```python
from build123d import *

# Parameters (mm, degrees)
SKETCH1_W                      = 95
SKETCH1_H                      = 34
BOSS_EXTRUDE1_DEPTH            = 6.5
SKETCH2_W                      = 74
SKETCH2_H                      = 5
BOSS_EXTRUDE2_DEPTH            = 90
SKETCH3_W                      = 58
SKETCH3_H                      = 22
CUT_EXTRUDE1_DEPTH             = 90
CBORE_FOR_M3_SHCS1_D           = 3.4
CBORE_FOR_M3_SHCS1_DEPTH       = 10.1
CBORE_FOR_M3_SHCS1_CBORE_D     = 6.5
CBORE_FOR_M3_SHCS1_CBORE_DEPTH = 3
CBORE_FOR_M3_SHCS1_TIP         = 1.021463052
SKETCH7_W                      = 6
SKETCH7_H                      = 20
BOSS_EXTRUDE3_DEPTH            = 20
CHAMFER1_SIZE                  = 20
F_1_0_3_5_DIAMETER_HOLE1_D     = 3.5
F_1_0_3_5_DIAMETER_HOLE1_DEPTH = 10.1
F_1_0_3_5_DIAMETER_HOLE1_TIP   = 1.051506083
SKETCH12_W                     = 35.5
SKETCH12_H                     = 90
CUT_EXTRUDE2_DEPTH             = 20
CHAMFER2_SIZE                  = 10
FILLET1_R                      = 10


# Some blends are built 0.0001 mm under size
with BuildPart() as part:
    # Sketch1 → Boss-Extrude1 (new body)
    with BuildSketch(Plane.XY):
        Rectangle(SKETCH1_W, SKETCH1_H)
    extrude(amount=BOSS_EXTRUDE1_DEPTH)

    # Sketch2 → Boss-Extrude2 (add)
    with BuildSketch(Plane(origin=(0, 0, 0), x_dir=(-1, 0, 0), z_dir=(0, 0, -1))):
        with Locations((0, -14.5)):
            Rectangle(SKETCH2_W, SKETCH2_H)
    extrude(amount=BOSS_EXTRUDE2_DEPTH)

    # Sketch3 → Cut-Extrude1 (cut)
    with BuildSketch(Plane(origin=(0, 0, 0), x_dir=(-1, 0, 0), z_dir=(0, 0, -1))):
        with Locations((0, -1)):
            Rectangle(SKETCH3_W, SKETCH3_H)
    extrude(amount=-CUT_EXTRUDE1_DEPTH, mode=Mode.SUBTRACT)

    # CBORE for M3 SHCS1
    with Locations(Plane.XY.offset(6.5)):
        with Locations((-43.42, 10), (-43.42, -10), (43.42, 10), (43.42, -10)):
            CounterBoreHole(CBORE_FOR_M3_SHCS1_D / 2, CBORE_FOR_M3_SHCS1_CBORE_D / 2, CBORE_FOR_M3_SHCS1_CBORE_DEPTH, depth=CBORE_FOR_M3_SHCS1_DEPTH)
            with Locations((0, 0, -(CBORE_FOR_M3_SHCS1_DEPTH + CBORE_FOR_M3_SHCS1_TIP / 2))):  # 118° drill point
                Cone(0, CBORE_FOR_M3_SHCS1_D / 2, CBORE_FOR_M3_SHCS1_TIP, mode=Mode.SUBTRACT)

    # Sketch7 → Boss-Extrude3 (add)
    with BuildSketch(Plane(origin=(0, 0, 0), x_dir=(-1, 0, 0), z_dir=(0, 0, -1))):
        with Locations((-34, -2)):
            Rectangle(SKETCH7_W, SKETCH7_H)
        with Locations((34, -2)):
            Rectangle(SKETCH7_W, SKETCH7_H)
    extrude(amount=BOSS_EXTRUDE3_DEPTH)

    # Chamfer1
    chamfer1_edges = [part.edges().sort_by_distance(p)[0] for p in [
        (34, 8, -20),
        (-34, 8, -20),
    ]]
    chamfer(chamfer1_edges, length=CHAMFER1_SIZE - 0.0001)  # a hair under: the kernel refuses the full size

    # Ø1.0 (3.5) Diameter Hole1
    with Locations(Plane(origin=(0, -12, 0), x_dir=(1, 0, 0), z_dir=(0, 1, 0))):
        with Locations((-24.5, 77), (24.5, 77), (-24.5, 19), (24.5, 19)):
            Hole(F_1_0_3_5_DIAMETER_HOLE1_D / 2, depth=F_1_0_3_5_DIAMETER_HOLE1_DEPTH)
            with Locations((0, 0, -(F_1_0_3_5_DIAMETER_HOLE1_DEPTH + F_1_0_3_5_DIAMETER_HOLE1_TIP / 2))):  # 118° drill point
                Cone(0, F_1_0_3_5_DIAMETER_HOLE1_D / 2, F_1_0_3_5_DIAMETER_HOLE1_TIP, mode=Mode.SUBTRACT)

    # Sketch12 → Cut-Extrude2 (cut)
    with BuildSketch(Plane(origin=(0, -12, 0), x_dir=(1, 0, 0), z_dir=(0, 1, 0))):
        with Locations((0, 45)):
            Rectangle(SKETCH12_W, SKETCH12_H)
    extrude(amount=-CUT_EXTRUDE2_DEPTH, mode=Mode.SUBTRACT)

    # Chamfer2
    chamfer2_edges = [part.edges().sort_by_distance(p)[0] for p in [
        (17.75, -14.5, 0),
        (-17.75, -14.5, 0),
        (37, -14.5, -90),
        (-37, -14.5, -90),
    ]]
    chamfer(chamfer2_edges, length=CHAMFER2_SIZE)

    # Fillet1
    # the kernel refuses this fillet: 10 mm, written as the material it takes off along each edge
    with BuildSketch(Plane(origin=(-17.75, 12.929588344, -90), x_dir=(0, 0, 1), z_dir=(0, -1, 0))) as fillet1_piece_1:
        with BuildLine():
            CenterArc((9.971835338, 10), FILLET1_R, 184.301222305, 85.698777695)
            Line((0, 9.25), (-0.199436707, 9.235))
            ThreePointArc((-0.199436707, 9.235), (-0.2, 4.625), (-0.2, 0))
            Line((-0.2, 0), (0, -0.2))
            Line((0, -0.2), (9.971835338, -0.2))
            Line((9.971835338, -0.2), (9.971835338, 0))
        make_face()
    extrude(amount=54.859176688, mode=Mode.SUBTRACT)
    with BuildSketch(Plane(origin=(17.75, 12.929588344, -90), x_dir=(1, 0, 0), z_dir=(0, -1, 0))) as fillet1_piece_2:
        with BuildLine():
            CenterArc((10, 9.971835338), FILLET1_R, 180, 85.698777695)
            Line((0, 9.971835338), (-0.2, 9.971835338))
            Line((-0.2, 9.971835338), (-0.2, 0))
            Line((-0.2, 0), (0, -0.2))
            ThreePointArc((0, -0.2), (4.625, -0.2), (9.235, -0.199436707))
            Line((9.235, -0.199436707), (9.25, 0))
        make_face()
    extrude(amount=54.859176688, mode=Mode.SUBTRACT)


solid = part.part
```
Geometry check sheet. Reference: the model listing, model coordinates, mm. A direction names the side the tool comes from. Coordinates: 2 decimals unless noted, no trailing zeros. Order: outer loops, then holes, each group sorted by start corner. A loop starts at its lowest first (then second) coordinate and runs counter-clockwise, first axis right, second up.
Q1. Sectioned sample at C-C on y = 5.5. Record the cut outline in (x, z), and give its area (3 significant figures).
Reply:
outline: (-47.5, 0) - (-37, 0) - (-37, -2.5) - (-31, -2.5) - (-31, 0) - (-29, 0) - (-29, 6.5) - (-47.5, 6.5) - close; (29, 0) - (31, 0) - (31, -2.5) - (37, -2.5) - (37, 0) - (47.5, 0) - (47.5, 6.5) - (29, 6.5) - close
area: 271 mm2
Q2. Tool access check on faces 4 (the face through (42.997, 13.222, 5.021)), 5 (the face through (17.75, -14, -45)), 6 (the face through (37, -13, -28)). Record the directions out of +Z, -Z, +X, -X, +Y, -Y that give a thin tool (end or side, any length) a straight path to the whole face; none if there is none.
Reply:
face 4: +Z
face 5: -Z, +Y, -Y
face 6: -Z, +X, +Y, -Y
Q3. Depth check by flat-ended pin: pin 1 Ø5 at (x, y) = (-43.42, 10) entering from +Z; pin 2 Ø5 at (x, y) = (-43.42, -10) entering from -Z; pin 3 Ø4 at (x, z) = (-24.5, -77) entering from +Y; pin 4 Ø22 at (x, z) = (1.5, -27) entering from +Y. Enter the tip coordinate at first touch or a pass-through.
Reply:
pin 1: stops at z = 3.5
pin 2: stops at z = 0
pin 3: stops at y = -12
pin 4: passes through
Q4. Draft check along Y on faces 1 (the face through (-47.5, 0, 3)), 2 (the face through (34, -2, -10)), 3 (the face through (-42, -11.4, 3.5)). Enter one of: released by +Y, released by -Y, zero draft, split by the parting line, or undercut.
Reply:
face 1: zero draft
face 2: released by +Y
face 3: undercut
Q5. Sectioned sample at A-A on x = 6. Record the cut outline in (y, z), and give its area (3 significant figures).
Reply:
outline: (-17, 0) - (-12, 0) - (-12, 6.5) - (-17, 6.5) - close; (10, 0) - (17, 0) - (17, 6.5) - (10, 6.5) - close
area: 78.0 mm2
Q6. Thickness scan on probe 1 along Y at (x, z) = (-43.42, 0.7); probe 2 along X at (y, z) = (-14, -19); probe 3 along Z at (x, y) = (24.5, -14). Record the ranges inside material, lowest first.
Reply:
probe 1: y = -17 to -11.7, -8.3 to 8.3, 11.7 to 17
probe 2: x = -37 to -26.25, -22.75 to -17.75, 17.75 to 22.75, 26.25 to 37
probe 3: z = -89.49 to -78.75, -75.25 to -20.75, -17.25 to 6.5
Q7. Sectioned sample at D-D on z = -54. Record the cut outline in (x, y).
Reply:
outline: (-37, -17) - (-17.75, -17) - (-17.75, -12) - (-37, -12) - close; (17.75, -17) - (37, -17) - (37, -12) - (17.75, -12) - close
Q8. Sectioned sample at B-B on z = -77. Record the cut outline in (x, y).
Reply:
outline: (-37, -17) - (-26.25, -17) - (-26.25, -12) - (-37, -12) - close; (-22.75, -17) - (-17.75, -17) - (-17.75, -12) - (-22.75, -12) - close; (17.75, -17) - (22.75, -17) - (22.75, -12) - (17.75, -12) - close; (26.25, -17) - (37, -17) - (37, -12) - (26.25, -12) - close
